The listing builds one solid part. Answer for the finished solid, in the listing's coordinates (mm). A direction names the side the tool comes from. Coordinates: 2 decimals unless noted, no trailing zeros. Order: outer loops, then holes, each group sorted by start corner. A loop starts at its lowest first (then second) coordinate and runs counter-clockwise, first axis right, second up. Notation, with made-up numbers: (81.5, -35) - (127.5, -35) arc R28 cw to (127.5, 0) - close; hole circle Ø2 at (14.25, -33.75). An arc over 180 degrees is marked (long way). Use one line per item in the form item = value. Start each with the question number.
Item 1: Section A-A, the plane y = 1.25 is taken. Write down the section's boundary in (x, z).
Item 2: The mould has two halves that part along Z. Classify faces 1 (the flat face through (14, 5, 9)), 2 (the cylindrical face through (22.968, 0.986, 15.843)), 3 (the flat face through (16, 3, -1.308)), 4 (the flat face through (-22, 3, 7.428)): released by +Z, released by -Z, zero draft, split by the parting line, or undercut.
Item 3: A tool of negligible diameter and unlimited length cuts with its end or side. For faces 5 (the flat face through (-27.789, 3, -4)), 6 (the flat face through (-17.92, 3, 6)), 7 (the flat face through (16, 3, -12.116)), 8 (the flat face through (-11.631, 3, -7)), from which of +Z, -Z, +X, -X, +Y, -Y can it reach the whole face along a straight path? Write none if from no direction.
Item 4: Section C-C, the plane z = -4.5 is taken. Write down the section's boundary in (x, y), and give its area (3 significant figures).
Item 5: Section B-B, the plane x = 25 is taken. Write down the section's boundary in (y, z).
Item 6: Section D-D, the plane y = 4.4 is taken. Write down the section's boundary in (x, z), and give its area (3 significant figures).
Item 7: Each of these flat-tipped pins is pushed along its axis until it touches: pin 1 Ø1.5 at (x, y) = (-8.5, 3) entering from -Z; pin 2 Ø1.5 at (y, z) = (3.5, 5.5) entering from -X; pin 3 Ø0.9 at (x, y) = (-10, 4) entering from +Z; pin 4 Ø3 at (x, z) = (20.5, -3.5) entering from -Y. Where does it stop, or does it pass through?
Item 8: Consider line 1 along X through (y, z) = (0.55, -15); line 2 along Z through (x, y) = (-25, 0.5); line 3 along Z through (x, y) = (1.5, 4.1). Determine where each line is inside the solid, lowest interval first. Write a range as [from, to].
from build123d import *

# Parameters (mm, degrees)
SKETCH1_W                  = 60
SKETCH1_H                  = 40
BOSS_EXTRUDE1_DEPTH        = 2
SKETCH2_W                  = 12.326283063
SKETCH2_H                  = 8.575111395
SKETCH2_W_2                = 13.737384573
SKETCH2_H_2                = 10.808942535
SKETCH2_W_3                = 18.592828035
SKETCH2_H_3                = 16.842728436
SKETCH2_W_4                = 7.411585369
SKETCH2_H_4                = 3.471203566
SKETCH2_W_5                = 14.654892662
SKETCH2_H_5                = 11.51389599
SKETCH2_W_6                = 18.043574534
SKETCH2_H_6                = 10.748392007
BOSS_EXTRUDE2_DEPTH        = 3
F_4_4_4_4_DIAMETER_HOLE1_D = 4.4


with BuildPart() as part:
    # Sketch1 → Boss-Extrude1 (new body)
    with BuildSketch(Plane(origin=(0, 0, 0), x_dir=(1, 0, 0), z_dir=(0, 1, 0))):
        Rectangle(SKETCH1_W, SKETCH1_H)
    extrude(amount=BOSS_EXTRUDE1_DEPTH)

    # Sketch2 → Boss-Extrude2 (add)
    with BuildSketch(Plane(origin=(0, 2, 0), x_dir=(1, 0, 0), z_dir=(0, 1, 0))):
        with Locations((-21.625666124, 4.358295229)):
            Rectangle(SKETCH2_W, SKETCH2_H)
        with Locations((16.207165307, 6.711999232)):
            Rectangle(SKETCH2_W_2, SKETCH2_H_2)
        with Locations((-2.33436777, 6.711999232)):
            Rectangle(SKETCH2_W_3, SKETCH2_H_3)
        with Locations((-21.625666124, -5.692081798)):
            Rectangle(SKETCH2_W_4, SKETCH2_H_4)
        with Locations((14.346591679, -9.340896656)):
            Rectangle(SKETCH2_W_5, SKETCH2_H_5)
        with Locations((-6.403086195, -11.066277802)):
            Rectangle(SKETCH2_W_6, SKETCH2_H_6)
    extrude(amount=BOSS_EXTRUDE2_DEPTH)

    # Ø4.4 (4.4) Diameter Hole1 (through all)
    with Locations(Plane(origin=(0, 2, 0), x_dir=(1, 0, 0), z_dir=(0, 1, 0))):
        with Locations((-25, 15), (25, 15), (25, -15), (-25, -15)):
            Hole(F_4_4_4_4_DIAMETER_HOLE1_D / 2)


solid = part.part
Response:
q1.outline = (-30, -20) - (30, -20) - (30, 20) - (-30, 20) - close; hole circle Ø4.4 at (-25, -15); hole circle Ø4.4 at (-25, 15); hole circle Ø4.4 at (25, -15); hole circle Ø4.4 at (25, 15)
q2.face_1 = zero draft
q2.face_2 = undercut
q2.face_3 = undercut
q2.face_4 = released by +Z
q3.face_5 = +Z, -Z, -X, +Y
q3.face_6 = +Z, +Y
q3.face_7 = -Z, +X, +Y
q3.face_8 = -Z, +Y
q4.outline = (-30, 0) - (30, 0) - (30, 2) - (23.08, 2) - (23.08, 5) - (9.34, 5) - (9.34, 2) - (6.96, 2) - (6.96, 5) - (-11.63, 5) - (-11.63, 2) - (-15.46, 2) - (-15.46, 5) - (-27.79, 5) - (-27.79, 2) - (-30, 2) - close
q4.area = 254 mm2
q5.outline = (0, -20) - (2, -20) - (2, -17.2) - (0, -17.2) - close; (0, -12.8) - (2, -12.8) - (2, 12.8) - (0, 12.8) - close; (0, 17.2) - (2, 17.2) - (2, 20) - (0, 20) - close
q6.outline = (-27.79, -8.65) - (-15.46, -8.65) - (-15.46, -0.07) - (-27.79, -0.07) - close; (-25.33, 3.96) - (-17.92, 3.96) - (-17.92, 7.43) - (-25.33, 7.43) - close; (-15.42, 5.69) - (2.62, 5.69) - (2.62, 16.44) - (-15.42, 16.44) - close; (-11.63, -15.13) - (6.96, -15.13) - (6.96, 1.71) - (-11.63, 1.71) - close; (7.02, 3.58) - (21.67, 3.58) - (21.67, 15.1) - (7.02, 15.1) - close; (9.34, -12.12) - (23.08, -12.12) - (23.08, -1.31) - (9.34, -1.31) - close
q6.area = 956 mm2
q7.pin_1 = -15.13
q7.pin_2 = -25.33
q7.pin_3 = 16.44
q7.pin_4 = 0
q8.line_1 = [-30, -27.2], [-22.8, 22.8], [27.2, 30]
q8.line_2 = [-20, -17.2], [-12.8, 12.8], [17.2, 20]
q8.line_3 = [-15.13, 1.71], [5.69, 16.44]
